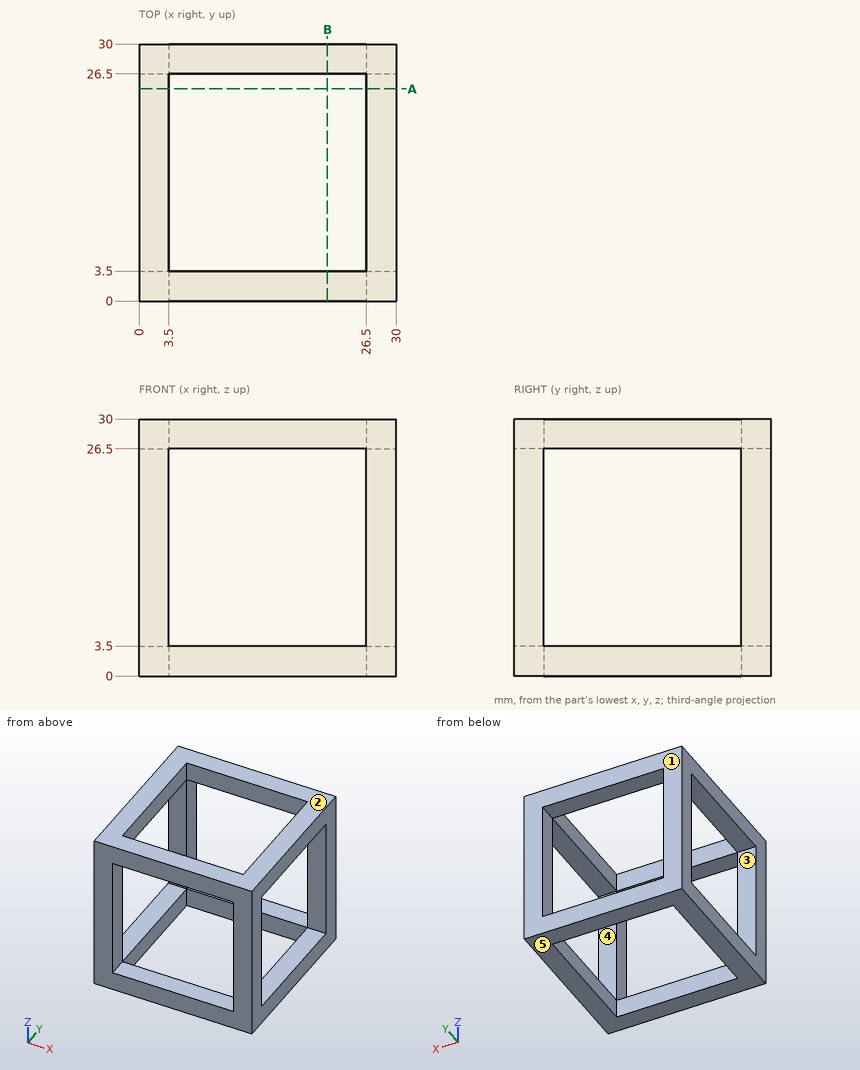
Source: three-view drawing plus pictorial views. Frame: mm from the lowest corner of the part. A direction names the side the tool comes from. Give positions to 0.01 mm unless a question says otherwise; leave off trailing zeros. Order: outer loops, then holes, each group sorted by start corner. A loop starts at its lowest first (then second) coordinate and runs counter-clockwise, first axis right, second up. Notation, with made-up numbers: M -12,51 L -1,51 A11 ccw -1,65 Z; hole C 89.25,-13 d10. An arc over 180 degrees is marked long. One line per question, with ' | ' between items. Start each with the question number.
1. Section query A-A (y = 24.75). Return the cut outline in (x, z), and give its area (3 significant figures).
2. Material intervals for probe 1 along X at (y, z) = (8.25, 2.5), sorted ascending. Write a range as [from, to].
3. Access query for the marked faces 4 and 5. Directions: +Z, -Z, +X, -X, +Y, -Y. A direction counts if a zero-diameter tool reaches every point of the face in a straight line with its end or side. Return the directions, or none.
4. Pull-direction query (Z, two-part tool) for the marked faces 1, 2 and 3; classes: released by +Z, released by -Z, zero draft, split by the parting line, or undercut.
Here are the results:
1) outline: M 0,0 L 3.5,0 L 3.5,3.5 L 0,3.5 Z; M 0,26.5 L 3.5,26.5 L 3.5,30 L 0,30 Z; M 26.5,0 L 30,0 L 30,3.5 L 26.5,3.5 Z; M 26.5,26.5 L 30,26.5 L 30,30 L 26.5,30 Z | area: 49.0 mm²
2) probe 1: [0, 3.5], [26.5, 30]
3) face 4: +X, -X | face 5: -Z, +X, -X, +Y, -Y
4) face 1: zero draft | face 2: released by +Z | face 3: undercut
